```python
from build123d import *

# Parameters (mm, degrees)
SKETCH1_R           = 90
SKETCH1_R_2         = 80
EXTRUDE_THIN1_DEPTH = 3
SKETCH2_W           = 45
SKETCH2_H           = 5
BOSS_EXTRUDE1_DEPTH = 20
CUT_EXTRUDE1_DEPTH  = 5
CIRPATTERN1_COUNT   = 6
SCALE1_SCALE        = 1.25


with BuildPart() as part:
    # Sketch1 → Extrude-Thin1 (new body)
    with BuildSketch(Plane(origin=(0, 0, 0), x_dir=(1, 0, 0), z_dir=(0, 1, 0))):
        Circle(SKETCH1_R)
        Circle(SKETCH1_R_2, mode=Mode.SUBTRACT)
    extrude(amount=EXTRUDE_THIN1_DEPTH)

    # Sketch2 → Boss-Extrude1 (add)
    with BuildSketch(Plane(origin=(0, 3, 0), x_dir=(1, 0, 0), z_dir=(0, 1, 0))):
        with Locations((67.465271077, 0)):
            Rectangle(SKETCH2_W, SKETCH2_H)
    boss_extrude1 = extrude(amount=BOSS_EXTRUDE1_DEPTH)

    # Sketch3 → Cut-Extrude1 (cut)
    with BuildSketch(Plane.XY.offset(2.5)):
        Polygon((44.965271077, 11.022693862), (72.510497513, 23), (44.965271077, 23), align=None)
    cut_extrude1 = extrude(amount=-CUT_EXTRUDE1_DEPTH, mode=Mode.SUBTRACT)

    # CirPattern1: Boss-Extrude1, Cut-Extrude1 ×6 about axis
    cirpattern1_axis = Axis((0, 0, 0), (0, 1, 0))
    for i in range(1, CIRPATTERN1_COUNT):
        add(boss_extrude1.rotate(cirpattern1_axis, i * 360 / CIRPATTERN1_COUNT))
        add(cut_extrude1.rotate(cirpattern1_axis, i * 360 / CIRPATTERN1_COUNT), mode=Mode.SUBTRACT)


with BuildPart() as part_1:
    # Scale1: scaled about (0, 7.379680738, 0)
    add(part.part.scale(SCALE1_SCALE).moved(Location((0, -1.844920185, 0))))


solid = part_1.part
```
CAD build for the part. Positions are in the model's coordinates, mm. A direction names the side the tool comes from. Round coordinates to 2 decimals unless told otherwise and drop trailing zeros. Order: outer loops, then holes, each group sorted by start corner. A loop starts at its lowest first (then second) coordinate and runs counter-clockwise, first axis right, second up. Notation, with made-up numbers: (-27, 18.5) - (-20, 18.5) arc R26 ccw to (-20, 55.5) - close; hole circle Ø8 at (53, 82.5). An arc over 180 degrees is marked (long way). Use CSV: the item, a comma, the result in double quotes. Start each with the question number.
1) Tool access for faces 1 (the flat face through (36.629, 19.314, -63.355)), 2 (the flat face through (42.39, 11.45, -79.67)), 3 (the flat face through (-28.065, 6.849, -48.698)): list every direction of +Z, -Z, +X, -X, +Y, -Y with a clear straight run to the whole face (end or side of a thin tool).
2) Saw through at A-A (x = 0). List the corners of the cut face in (y, z), and give its area (4 significant figures).
3) Wall check: L1, parallel to X at y = 9.5, z = 0; L2, parallel to X at y = 1.05, z = 0; L3, parallel to Y at x = -95.5, z = 36. Give the ranges that are in metal, low to high. Write a range as [from, to].
4) Pin check, flat tips, straight feed: pin 1 Ø12 at (y, z) = (16.5, -38.5) entering from -X; pin 2 Ø22 at (x, z) = (40, 66.5) entering from -Y; pin 3 Ø1.9 at (y, z) = (16.5, -1.5) entering from -X; pin 4 Ø12.5 at (x, y) = (88, 18) entering from -Z (3 decimals). Stop position of each tip, or through.
5) Saw through at B-B (z = 0). List the corners of the cut face in (x, y), and give its area (3 significant figures).
6) Two-plate mould, pull along X, no slides. Class faces 4 (the flat face through (47.8, 11.45, 76.54)), 5 (the flat face through (89, 1.905, 49)), 6 (the flat face through (-73.181, 19.314, -0.044)): pulls with the +X half, pulls with the -X half, needs draft (parallel to the pull), parting line crosses it, or undercut.
7) Saw through at C-C (y = 17). List the corners of the cut face in (x, z) (3 decimals).
8) Saw through at D-D (x = 84.5). List the corners of the cut face in (y, z) (3 decimals), and give its area (3 significant figures).
Values follow:
1,face 1,"+Y"
1,face 2,"-Z, +Y"
1,face 3,"+Y, -Y"
2,outline,"(-1.84, -112.5) - (1.91, -112.5) - (1.91, -100) - (-1.84, -100) - close; (-1.84, 100) - (1.91, 100) - (1.91, 112.5) - (-1.84, 112.5) - close"
2,area,"93.75 mm2"
3,L1,"x = [-112.46, -56.21], [56.21, 112.46]"
3,L2,"x = [-112.5, -100], [100, 112.5]"
3,L3,"y = [-1.84, 1.91]"
4,pin 1,"passes through"
4,pin 2,"stops at y = 1.91"
4,pin 3,"stops at x = -112.46"
4,pin 4,"stops at z = -3.125"
5,outline,"(-112.5, -1.84) - (-100, -1.84) - (-100, 1.91) - (-56.21, 1.91) - (-56.21, 11.93) - (-90.64, 26.91) - (-112.46, 26.91) - (-112.46, 1.91) - (-112.5, 1.91) - close; (56.21, 1.91) - (100, 1.91) - (100, -1.84) - (112.5, -1.84) - (112.5, 1.91) - (112.46, 1.91) - (112.46, 26.91) - (90.64, 26.91) - (56.21, 11.93) - close"
5,area,"2,390 mm2"
6,face 4,"pulls with the +X half"
6,face 5,"needs draft"
6,face 6,"undercut"
7,outline,"(-112.457, -3.125) - (-67.859, -3.125) - (-67.859, 3.125) - (-112.457, 3.125) - close; (-58.935, -95.828) - (-53.522, -98.953) - (-31.223, -60.33) - (-36.636, -57.205) - close; (-58.935, 95.828) - (-36.636, 57.205) - (-31.223, 60.33) - (-53.522, 98.953) - close; (31.223, -60.33) - (53.522, -98.953) - (58.935, -95.828) - (36.636, -57.205) - close; (31.223, 60.33) - (36.636, 57.205) - (58.935, 95.828) - (53.522, 98.953) - close; (67.859, -3.125) - (112.457, -3.125) - (112.457, 3.125) - (67.859, 3.125) - close"
8,outline,"(-1.845, -74.27) - (1.905, -74.27) - (1.905, -53.477) - (-1.845, -53.477) - close; (-1.845, 53.477) - (1.905, 53.477) - (1.905, 74.27) - (-1.845, 74.27) - close; (1.905, -3.125) - (24.236, -3.125) - (24.236, 3.125) - (1.905, 3.125) - close"
8,area,"296 mm2"
